Part model, mm, in its own coordinate system. A direction names the side the tool comes from. Coordinates: 2 decimals unless noted, no trailing zeros. Order: outer loops, then holes, each group sorted by start corner. A loop starts at its lowest first (then second) coordinate and runs counter-clockwise, first axis right, second up.
Autodesk Inventor part; units mm, degrees
ref_plane "Work Plane1" through (0, 0, -9) normal (0, 0, -1) x (-1, 0, 0)
ref_plane "YZ Plane" through (0, 0, 0) normal (1, 0, 0) x (0, 1, 0)
ref_plane "XZ Plane" through (0, 0, 0) normal (0, 1, 0) x (-1, 0, 0)
sketch "Sketch1" plane through (0, 0, 0) normal (0, 0, 1) x (1, 0, 0)
  circle A0 centre (0, 0) radius 2.5
  arc A1 (0, 10) -> (0, -10) centre (0, 0) ccw
  line L0 (0, 10) -> (12, 10)
  line L1 (0, -10) -> (12, -10)
  line L2 (12, -10) -> (12, 10)
  dimension "d0" = 5
  dimension "d1" = 20
  dimension "d2" = 12
extrude "Extrusion1" add sketch "Sketch1" along normal blind 2
sketch "Sketch5" plane through (0, 0, 0) normal (0, 0, -1) x (-1, 0, 0)
  circle A0 centre (0, 0) radius 2.5
  line L0 (-12, -10) -> (0, -10)
  line L1 (0, -10) -> (0, -8)
  line L2 (0, -8) -> (-12, -8)
  line L3 (-12, -8) -> (-12, -10)
  line L4 (-12, 10) -> (-1, 10)
  line L5 (-1, 10) -> (-1, 8)
  line L6 (-1, 8) -> (-12, 8)
  line L7 (-12, 8) -> (-12, 10)
  dimension "d21" = 2
  dimension "d22" = 2
  dimension "d24" = 1
extrude "Extrusion5" add sketch "Sketch5" along normal blind 2 contours L3 L2 L1 L0 | L4 L5 L6 L7
sketch "Sketch6" plane through (0, 0, -2) normal (0, 0, -1) x (-1, 0, 0)
  line L0 (-12, 8) -> (-1, 8)
  line L1 (-1, 8) -> (-1, 10)
  line L2 (-1, 9.162) -> (-2.5994, 8)
  line L3 (-2.5994, 8) -> (6.8052, -4.9443) construction
  line L4 (6.8052, -4.9443) -> (8.4046, -3.7823) construction
  line L5 (8.4046, -3.7823) -> (-1, 9.162) construction
  line L6 (-2.5994, 8) -> (-1, 8)
  line L7 (-1, 9.162) -> (-1, 8)
  point P0 (0, 0)
  dimension "d27" = 16
  dimension "d28" = 8
  dimension "d29" = 36
extrude "Extrusion6" cut sketch "Sketch6" against normal blind 2
ref_plane "Work Plane1" through (0, 0, -9) normal (0, 0, -1) x (-1, 0, 0)
mirror "Mirror1" about plane through (0, 0, -9) normal (0, 0, -1)
sketch "Sketch7" plane through (0, -10, -16) normal (0, 0, 1) x (1, 0, 0)
  line L0 (12, 0) -> (0, 0)
  line L1 (12, 2) -> (12, 0)
  line L2 (0, 2) -> (12, 2)
  line L3 (0, 0) -> (0, 2)
  line L4 (2.5994, 18) -> (1, 19.162)
  line L5 (12, 18) -> (2.5994, 18)
  line L6 (12, 20) -> (12, 18)
  line L7 (1, 20) -> (12, 20)
  line L8 (1, 19.162) -> (1, 20)
  point P0 (0, 10)
extrude "Extrusion7" add sketch "Sketch7" along normal blind 14
sketch "Sketch8" plane through (12, -10, 2) normal (1, 0, 0) x (0, 0, -1)
  line L0 (22, 20) -> (0, 20)
  line L1 (0, 0) -> (0, 20)
  line L2 (22, 0) -> (0, 0)
  line L3 (22, 0) -> (22, 20)
  line L4 (2, 18) -> (20, 18)
  line L5 (20, 2) -> (20, 18)
  line L6 (2, 2) -> (20, 2)
  line L7 (2, 2) -> (2, 18)
  point P0 (2, 10)
extrude "Extrusion8" add sketch "Sketch8" along normal blind 20
sketch "Sketch9" plane through (0, 0, -20) normal (0, 0, -1) x (-1, 0, 0)
  line L0 (-32, 10) -> (0, 10)
  line L1 (-32, -10) -> (-32, 10)
  line L2 (-32, -6) -> (-12, 10)
  dimension "d37" = 20
  dimension "d38" = 4
extrude "Extrusion9" cut sketch "Sketch9" against normal blind 22
sketch "Sketch10" plane through (0, -8, 0) normal (0, 1, 0) x (1, 0, 0)
  line L0 (32, 0) -> (0, 0)
  line L1 (32, 18) -> (32, 0)
  line L2 (0, 18) -> (32, 18)
  line L3 (15, 15) -> (29, 15) construction
  line L4 (29, 15) -> (29, 3) construction
  line L5 (29, 3) -> (15, 3) construction
  line L6 (15, 3) -> (15, 15) construction
  circle A0 centre (15, 3) radius 1.6
  circle A1 centre (29, 3) radius 1.6
  circle A2 centre (29, 15) radius 1.6
  circle A3 centre (15, 15) radius 1.6
  dimension "d41" = 3.2
  dimension "d42" = 3
  dimension "d43" = 3
  dimension "d44" = 3
  dimension "d45" = 14
extrude "Extrusion10" cut sketch "Sketch10" against normal through all
properties part number "x_axis_cable_mount_a" material "ABS Plastic"
Q1. Cut at D-D on x = 29. Write the cut outline in (y, z), and give its area (3 significant figures).
Results list:
outline: (-10, -20) - (-3.6, -20) - (-3.6, -18) - (-8, -18) - (-8, -16.6) - (-10, -16.6) - close; (-10, -13.4) - (-8, -13.4) - (-8, -4.6) - (-10, -4.6) - close; (-10, -1.4) - (-8, -1.4) - (-8, 0) - (-3.6, 0) - (-3.6, 2) - (-10, 2) - close
area: 48.8 mm2
Q2. Pin check, flat tips, straight feed: pin 1 Ø6 at (y, z) = (1.5, -5) entering from -X; pin 2 Ø9 at (x, z) = (19.5, -10.5) entering from +Y; pin 3 Ø2 at (y, z) = (0, -17.5) entering from +X; pin 4 Ø1 at (y, z) = (-9, -11.5) entering from -X. Stop position of each tip, or through.
Results list:
pin 1: passes through
pin 2: stops at y = -8
pin 3: stops at x = 25.58
pin 4: stops at x = 0
Q3. Mould opens along X. For faces 1 (the face through (16, -10, -9)), 2 (the face through (1, 9.6, -8.9)), 3 (the face through (13.4, -8.99, -3.07)) say: pulls with the +X half, pulls with the -X half, needs draft (parallel to the pull), parting line crosses it, or undercut.
Results list:
face 1: needs draft
face 2: pulls with the -X half
face 3: undercut
Q4. Wall check: line 1 along Z through (x, y) = (29, -9.2); line 2 along X through (y, z) = (-9, -15); line 3 along Y through (x, z) = (8, -0.5). Give the ranges that are in metal, low to high.
Results list:
line 1: z = -20 to -16.6, -13.4 to -4.6, -1.4 to 2
line 2: x = 0 to 13.4, 16.6 to 27.4, 30.6 to 32
line 3: y = -10 to -8, 8 to 10
Q5. Cut at C-C on y = 0. Write the cut outline in (x, z).
Results list:
outline: (-10, -20) - (-2.5, -20) - (-2.5, -18) - (-10, -18) - close; (-10, 0) - (-2.5, 0) - (-2.5, 2) - (-10, 2) - close; (2.5, -20) - (24.5, -20) - (24.5, -18) - (2.5, -18) - close; (2.5, 0) - (24.5, 0) - (24.5, 2) - (2.5, 2) - close
Q6. Cut at A-A on x = 15. Write the cut outline in (y, z), and give its area (3 significant figures).
Results list:
outline: (-10, -20) - (7.6, -20) - (7.6, -18) - (-8, -18) - (-8, -16.6) - (-10, -16.6) - close; (-10, -13.4) - (-8, -13.4) - (-8, -4.6) - (-10, -4.6) - close; (-10, -1.4) - (-8, -1.4) - (-8, 0) - (7.6, 0) - (7.6, 2) - (-10, 2) - close
area: 93.6 mm2
Q7. Cut at B-B on z = -3. Write the cut outline in (x, y).
Results list:
outline: (0, -10) - (13.4, -10) - (13.4, -8) - (0, -8) - close; (1, 9.16) - (2.6, 8) - (14.5, 8) - (12, 10) - (1, 10) - close; (16.6, -10) - (27.4, -10) - (27.4, -8) - (16.6, -8) - close; (30.6, -10) - (32, -10) - (32, -8) - (30.6, -8) - close
Q8. Which spindle directions (+Z, -Z, +X, -X, +Y, -Y) get a long thin tool onto all of the face, cutting with end or side? Do faces 4 (the face through (0, -9, -9)), 5 (the face through (8, 8, -9)), 6 (the face through (1.79, 8.59, -9.13)). Say none if no direction does.
Results list:
face 4: -X, +Y, -Y
face 5: +X, -X
face 6: -X
